from build123d import *

# Parameters (mm, degrees)
F0_R     = 3.6
F0_R_2   = 3.1
F1_DEPTH = 12.5
F2_R     = 5
F3_DEPTH = 12.5
F5_DEPTH = 4
F6_R     = 5.6839494551
F6_R_2   = 3.6
F7_DEPTH = 25


# Not quite as in the source:
# - a feature names something its author has since deleted; it is built from what else it names


with BuildPart() as f1:
    # F0 (on Front) → F1 (new body, symmetric)
    with BuildSketch(Plane.XZ):
        Circle(F0_R)
        Circle(F0_R_2, mode=Mode.SUBTRACT)
    extrude(amount=F1_DEPTH, both=True)

    # F2 (on Top) → F3 (cut, symmetric)
    with BuildSketch(Plane.XY):
        with Locations((0, -16.1383841203)):
            Circle(F2_R)
    extrude(amount=F3_DEPTH, both=True, mode=Mode.SUBTRACT)

    # F4 (on Right) → F5 (join, symmetric)
    with BuildSketch(Plane.YZ):
        Polygon((-15.2992176846, -2.8184308636), (-15.0516938496, -3.2091679669), (-8.7361828689, 0.7915769966), (-8.9837067039, 1.1823140999), align=None)
    extrude(amount=F5_DEPTH, both=True)

    # F6 (on Front) → F7 (cut, symmetric)
    with BuildSketch(Plane.XZ):
        Circle(F6_R)
        Circle(F6_R_2, mode=Mode.SUBTRACT)
    extrude(amount=F7_DEPTH, both=True, mode=Mode.SUBTRACT)


solid = f1.part
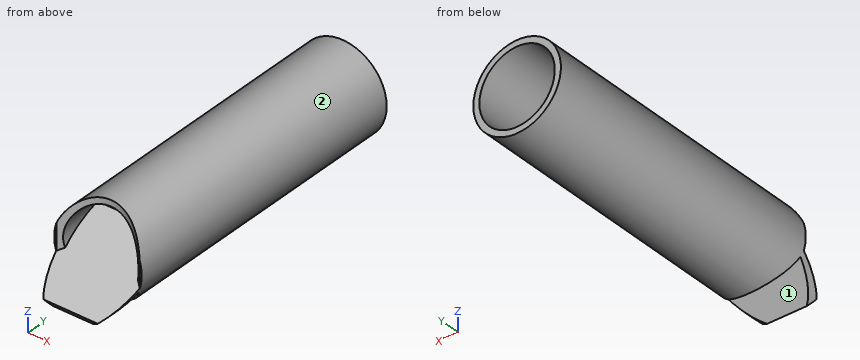
Design review of the part built by this model. Coordinates are the model's own, in mm. Face numbers are marked on the shaded views. Coordinates: 2 decimals unless noted, no trailing zeros. Loops run counter-clockwise (first coordinate to the right, second up) from the corner with the lowest first, then second, coordinate; pieces in that order, holes last. Notation, with made-up numbers: (77.5, 80) - (109.5, 80) arc R18 ccw to (109.5, 85) - close; hole circle Ø10 at (77.5, -18). An arc over 180 degrees is marked (long way). Use CSV: the item, a comma, the result in double quotes. Start each with the question number.
1. To check wall thickness, follow probe 1 along Z at (x, y) = (0, 1); probe 2 along Z at (x, y) = (2.5, -0.5). State the ranges of each line that lie inside material, in increasing order.
2. Add section B-B on z = 2.5. Give the boundary of the cut face in (x, y).
3. Mouldability with a two-part tool opening along Z and no side actions: class the marked faces 1 and 2 as released by +Z, released by -Z, zero draft, split by the parting line, or undercut.
4. Add section A-A on x = 0. Give the boundary of the cut face in (y, z).
5. Clearance check with flat-ended pins moving along their axes: pin 1 (3 mm diameter, centred on x = -0.5, z = 0.5, fed in from -Y); pin 2 (2 mm diameter, centred on x = -0.5, z = -1, fed in from -Y); pin 3 (1 mm diameter, centred on y = 2.5, z = -1.5, fed in from -X); pin 4 (3 mm diameter, centred on x = -0.5, y = 9.5, fed in from +Z). State where each tip first meets the part, or that it passes through.
6. Add section D-D on y = 10.5. Give the boundary of the cut face in (x, z), plus the area to 3 significant figures.
7. Add section C-C on z = -2. Give the boundary of the cut face in (x, y), plus the area to 3 significant figures.
Resolved:
1,probe 1,"-3.6 to -3.1, 3.1 to 3.6"
1,probe 2,"-2.59 to -1.83, 1.83 to 2.59"
2,outline,"(-2.59, -11.86) arc R5 cw to (-1.83, -11.49) - (-1.83, 12.5) - (-2.59, 12.5) - close; (1.83, -11.49) arc R5 cw to (2.59, -11.86) - (2.59, 12.5) - (1.83, 12.5) - close"
3,face 1,"undercut"
3,face 2,"split by the parting line"
4,outline,"(-15.3, -2.82) - (-15.05, -3.21) - (-8.74, 0.79) - (-8.98, 1.18) - close; (-11.14, -3.6) - (12.5, -3.6) - (12.5, -3.1) - (-11.14, -3.1) - close; (-11.14, 3.1) - (12.5, 3.1) - (12.5, 3.6) - (-11.14, 3.6) - close"
5,pin 1,"y = -12.43"
5,pin 2,"y = -14.01"
5,pin 3,"x = -3.46"
5,pin 4,"z = 3.6"
6,outline,"circle Ø7.2 at (0, 0); hole circle Ø6.2 at (0, 0)"
6,area,"10.5 mm2"
7,outline,"(-2.99, -14.01) - (2.99, -14.01) - (2.99, -13.14) - (-2.99, -13.14) - close; (-2.99, -12.13) arc R5 cw to (-2.37, -11.73) - (-2.37, 12.5) - (-2.99, 12.5) - close; (2.37, -11.73) arc R5 cw to (2.99, -12.13) - (2.99, 12.5) - (2.37, 12.5) - close"
7,area,"35.7 mm2"
